Study the drawing (mm; zero at the part's minimum x, y, z) and answer. A direction names the side the tool comes from. Give positions to 0.01 mm unless a question says otherwise; leave off trailing zeros. Order: outer loops, then holes, each group sorted by start corner. A loop starts at its lowest first (then second) coordinate and runs counter-clockwise, first axis right, second up. Notation, with made-up numbers: (9, 32) - (45, 32) arc R15 cw to (45, 44) - close; hole circle Ø5 at (-16, -6.75). An arc over 180 degrees is marked (long way). Write each question's results on one line, items separated by ' | '. Start each with the question number.
1. Which of the six approach directions +Z, -Z, +X, -X, +Y, -Y give full straight-line access (tool end or side, diameter ignored) to the marked faces 1 and 2?
2. Flat-ended cylindrical pins translate along their axes: pin 1 (2 mm diameter, centred on y = 44.5, z = 41, fed in from +X); pin 2 (17 mm diameter, centred on x = 44.5, z = 17, fed in from +Y); pin 3 (0.8 mm diameter, centred on x = 2, y = 20, fed in from -Z); pin 4 (12 mm diameter, centred on x = 62, y = 13, fed in from -Z). Find the tip coordinate at first contact, or state that the pin passes through.
3. Section A-A (x = 42) is taken. Give the vertices of the cut face in (y, z).
4. Section C-C (y = 37.5) is taken. Give the vertices of the cut face in (x, z).
5. Section D-D (z = 20) is taken. Give the vertices of the cut face in (x, y).
6. Section B-B (z = 40.5) is taken. Give the vertices of the cut face in (x, y) (3 decimals).
7. Find the intervals of material crossed by L1, parallel to Y at x = 0.85, z = 52 (3 decimals); L2, parallel to X at y = 1.85, z = 44 (3 decimals); L3, parallel to Z at x = 45.3, y = 0.9, in increasing order.
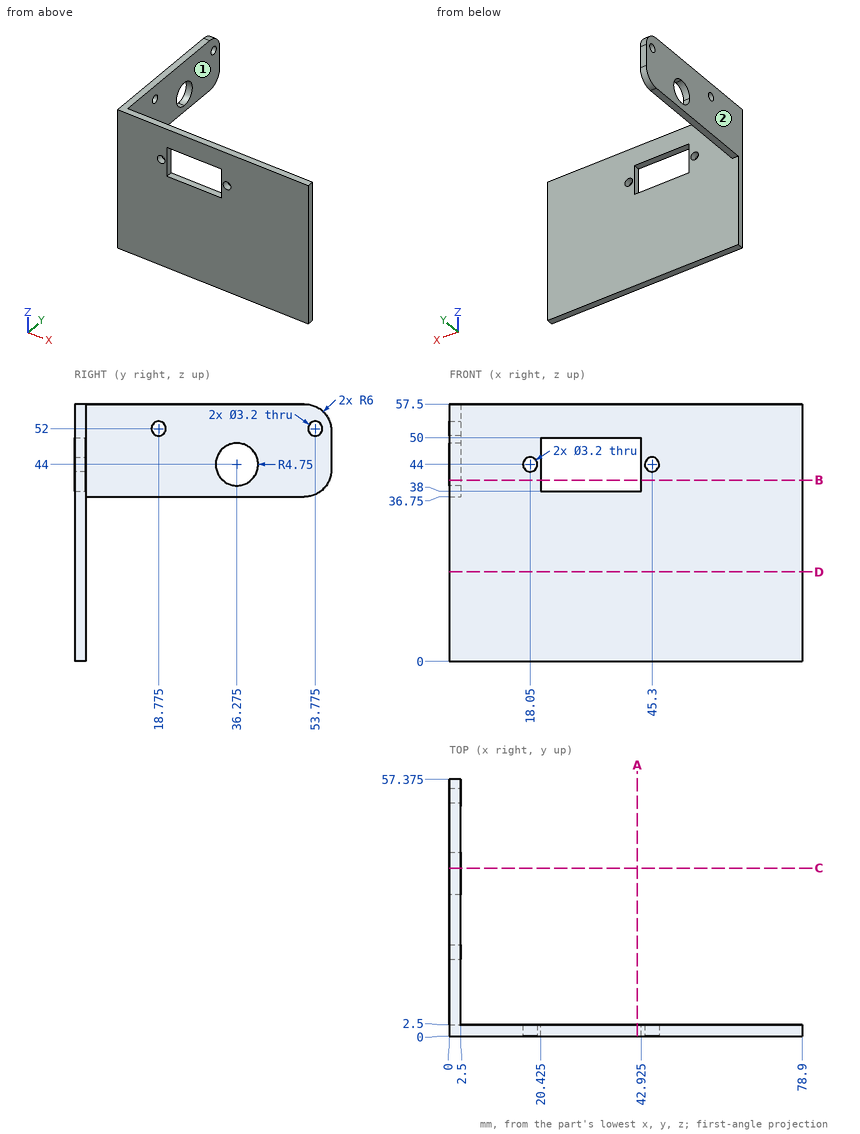
Reported:
1) face 1: +Z, -Z, +X, +Y | face 2: +Z, -Z, -X, +Y, -Y
2) pin 1: x = 2.5 | pin 2: y = 2.5 | pin 3: z = 36.75 | pin 4: through
3) outline: (0, 0) - (2.5, 0) - (2.5, 38) - (0, 38) - close; (0, 50) - (2.5, 50) - (2.5, 57.5) - (0, 57.5) - close
4) outline: (0, 36.75) - (2.5, 36.75) - (2.5, 39.41) - (0, 39.41) - close; (0, 48.59) - (2.5, 48.59) - (2.5, 57.5) - (0, 57.5) - close
5) outline: (0, 0) - (78.9, 0) - (78.9, 2.5) - (0, 2.5) - close
6) outline: (0, 0) - (20.425, 0) - (20.425, 2.5) - (2.5, 2.5) - (2.5, 33.064) - (0, 33.064) - close; (0, 39.486) - (2.5, 39.486) - (2.5, 56.937) - (0, 56.937) - close; (42.925, 0) - (78.9, 0) - (78.9, 2.5) - (42.925, 2.5) - close
7) L1: 0 to 17.175, 20.375 to 52.175, 55.375 to 57.354 | L2: 0 to 16.45, 19.65 to 20.425, 42.925 to 43.7, 46.9 to 78.9 | L3: 0 to 42.4, 45.6 to 57.5
